The listing builds one solid part. Answer for the finished solid, in the listing's coordinates (mm). A direction names the side the tool comes from. Give positions to 0.01 mm unless a question says otherwise; leave off trailing zeros. Order: outer loops, then holes, each group sorted by start corner. A loop starts at its lowest first (then second) coordinate and runs counter-clockwise, first axis right, second up. Notation, with made-up numbers: M -1,23.5 L 56,23.5 A15 ccw 56,35.5 Z; hole C 33,58.25 d5. An arc over 180 degrees is marked long. Answer as a JSON object with one key per item and string values. Group by question number.
```python
from build123d import *
from OCP.BRepFilletAPI import BRepFilletAPI_MakeChamfer

# Parameters (mm, degrees)
SKETCH1_W           = 10.16
SKETCH1_H           = 7.75
BOSS_EXTRUDE1_DEPTH = 10
CHAMFER1_SIZE       = 4
CHAMFER1_SIZE2      = 1.950930354
SKETCH2_R           = 1.6
CUT_EXTRUDE1_DEPTH  = 2
SKETCH3_W           = 4.58
SKETCH3_H           = 5.5
CUT_EXTRUDE2_DEPTH  = 1
SKETCH4_R           = 1.9
CUT_EXTRUDE3_DEPTH  = 5
SKETCH5_R           = 0.625
BOSS_EXTRUDE2_DEPTH = 3.5
CHAMFER2_SIZE       = 0.5
CHAMFER2_SIZE2      = 0.243866294


with BuildPart() as part:
    # Sketch1 → Boss-Extrude1 (new body)
    with BuildSketch(Plane.XY):
        Rectangle(SKETCH1_W, SKETCH1_H)
    extrude(amount=BOSS_EXTRUDE1_DEPTH)

    # Chamfer1
    chamfer1_edges = [part.edges().sort_by_distance(p)[0] for p in [
        (0, -3.875, 10),
    ]]
    chamfer1_side = [part.faces().sort_by_distance(p)[0] for p in [
        (0, -3.875, 5),
    ]]
    chamfer(chamfer1_edges, length=CHAMFER1_SIZE, length2=CHAMFER1_SIZE2, reference=chamfer1_side[0])

    # Sketch2 → Cut-Extrude1 (cut)
    with BuildSketch(Plane.XY.offset(10)):
        with Locations((-2.54, 0)):
            Circle(SKETCH2_R)
        with Locations((2.54, 0)):
            Circle(SKETCH2_R)
    extrude(amount=-CUT_EXTRUDE1_DEPTH, mode=Mode.SUBTRACT)

    # Sketch3 → Cut-Extrude2 (cut)
    with BuildSketch(Plane.XZ.offset(3.875)):
        with Locations((-2.54, 3)):
            Rectangle(SKETCH3_W, SKETCH3_H)
        with Locations((2.54, 3)):
            Rectangle(SKETCH3_W, SKETCH3_H)
    extrude(amount=-CUT_EXTRUDE2_DEPTH, mode=Mode.SUBTRACT)

    # Sketch4 → Cut-Extrude3 (cut)
    with BuildSketch(Plane.XZ.offset(2.875)):
        with Locations((-2.54, 2.5)):
            Circle(SKETCH4_R)
        with Locations((2.54, 2.5)):
            Circle(SKETCH4_R)
    extrude(amount=-CUT_EXTRUDE3_DEPTH, mode=Mode.SUBTRACT)

    # Sketch5 → Boss-Extrude2 (add)
    with BuildSketch(Plane(origin=(0, 0, 0), x_dir=(-1, 0, 0), z_dir=(0, 0, -1))):
        with Locations((2.54, 0)):
            Circle(SKETCH5_R)
        with Locations((-2.54, 0)):
            Circle(SKETCH5_R)
    extrude(amount=BOSS_EXTRUDE2_DEPTH)

    # Chamfer2: one chamfer whose edges measure the first distance from different faces: ONE call of the kernel's chamfer builder (chamfer() names one face for all edges)
    chamfer2_edges_1 = [part.edges().sort_by_distance(p)[0] for p in [
        (-1.915, 0, -3.5),
    ]]
    chamfer2_side_1 = [part.faces().sort_by_distance(p)[0] for p in [
        (-1.915, 0, -1.75),
    ]]
    chamfer2_edges_2 = [part.edges().sort_by_distance(p)[0] for p in [
        (3.165, 0, -3.5),
    ]]
    chamfer2_side_2 = [part.faces().sort_by_distance(p)[0] for p in [
        (3.165, 0, -1.75),
    ]]
    chamfer2 = BRepFilletAPI_MakeChamfer(part.part.solid().wrapped)
    for e in chamfer2_edges_1:
        chamfer2.Add(CHAMFER2_SIZE, CHAMFER2_SIZE2, e.wrapped, chamfer2_side_1[0].wrapped)  # the first distance lies on this face
    for e in chamfer2_edges_2:
        chamfer2.Add(CHAMFER2_SIZE, CHAMFER2_SIZE2, e.wrapped, chamfer2_side_2[0].wrapped)  # the first distance lies on this face
    add(Compound.cast(chamfer2.Shape()), mode=Mode.REPLACE)


solid = part.part
```
Item 1: Section D-D (y = 1.75) is taken. Determine the outline of the cut face in (x, z), and give its area (3 significant figures).
Item 2: Section C-C (x = -2.54) is taken. Determine the outline of the cut face in (y, z) (3 decimals), and give its area (3 significant figures).
Item 3: Section B-B (z = 2.5) is taken. Determine the outline of the cut face in (x, y) (3 decimals).
Item 4: Flat-ended cylindrical pins translate along their axes: P1, Ø1.1, axis at x = -3.5, y = -3.5, coming from the -Z side; P2, Ø1, axis at x = 2, y = 1, coming from the +Z side; P3, Ø3, axis at x = 2.54, z = 2.5, coming from the -Y side (3 decimals); P4, Ø0.5, axis at x = -3.5, y = -3.5, coming from the +Z side. Find the tip coordinate at first contact, or state that the pin passes through.
Item 5: Section A-A (y = 0) is taken. Determine the outline of the cut face in (x, z) (3 decimals), and give its area (3 significant figures).
Item 6: A tool of negligible diameter and unlimited length cuts with its end or side. For faces 1 (the flat face through (0, -3.875, 3)), 2 (the flat face through (2.5, -3.4, 0.25)), 3 (the flat face through (-3, 0, 8)), from which of +Z, -Z, +X, -X, +Y, -Y can it reach the whole face along a straight path? Write none if from no direction.
Item 7: Consider probe 1 along X at (y, z) = (-1, 3.25); probe 2 along X at (y, z) = (-1.75, 1); probe 3 along Z at (x, y) = (2.54, -0.9). Determine where each line is inside the solid, lowest interval first. Write a range as from..to.
Item 8: Determine the mould class of faces 4 (the flat face through (-0.1, -2.9, 8)), 5 (the cylindrical face through (-4.14, 0.07, 9.01)), 6 (the flat face through (-4.83, -3.4, 3)) for opening direction Z: released by +Z, released by -Z, zero draft, split by the parting line, or undercut.
Values found:
{
 "1": {"outline": "M -5.08,0 L 5.08,0 L 5.08,10 L -5.08,10 Z; hole C -2.54,2.5 d3.8; hole C 2.54,2.5 d3.8", "area": "78.9 mm^2"},
 "2": {"outline": "M -3.875,0 L -0.625,0 L -0.625,-3 L -0.381,-3.5 L 0.381,-3.5 L 0.625,-3 L 0.625,0 L 3.875,0 L 3.875,10 L 1.6,10 L 1.6,8 L -1.6,8 L -1.6,10 L -1.924,10 L -3.875,6 L -3.875,5.75 L -2.875,5.75 L -2.875,4.4 L 2.125,4.4 L 2.125,0.6 L -2.875,0.6 L -2.875,0.25 L -3.875,0.25 Z", "area": "47.0 mm^2"},
 "3": {"outline": "M -5.08,-3.875 L -4.83,-3.875 L -4.83,-2.875 L -4.44,-2.875 L -4.44,2.125 L -0.64,2.125 L -0.64,-2.875 L -0.25,-2.875 L -0.25,-3.875 L 0.25,-3.875 L 0.25,-2.875 L 0.64,-2.875 L 0.64,2.125 L 4.44,2.125 L 4.44,-2.875 L 4.83,-2.875 L 4.83,-3.875 L 5.08,-3.875 L 5.08,3.875 L -5.08,3.875 Z"},
 "4": {"P1": "stops at z = 0", "P2": "stops at z = 10", "P3": "stops at y = 2.125", "P4": "stops at z = 7.28"},
 "5": {"outline": "M -5.08,0 L -3.165,0 L -3.165,-3 L -2.921,-3.5 L -2.159,-3.5 L -1.915,-3 L -1.915,0 L 1.915,0 L 1.915,-3 L 2.159,-3.5 L 2.921,-3.5 L 3.165,-3 L 3.165,0 L 5.08,0 L 5.08,10 L 4.14,10 L 4.14,8 L 0.94,8 L 0.94,10 L -0.94,10 L -0.94,8 L -4.14,8 L -4.14,10 L -5.08,10 Z; hole C -2.54,2.5 d3.8; hole C 2.54,2.5 d3.8", "area": "74.6 mm^2"},
 "6": {"face 1": "+Z, -Z, +X, -X, -Y", "face 2": "-Y", "face 3": "+Z"},
 "7": {"probe 1": "x = -5.08..-4.29, -0.79..0.79, 4.29..5.08", "probe 2": "x = -5.08..-3.71, -1.37..1.37, 3.71..5.08", "probe 3": "z = 0..0.6, 4.4..8"},
 "8": {"face 4": "released by +Z", "face 5": "zero draft", "face 6": "undercut"}
}
